Study the drawing (mm; zero at the part's minimum x, y, z) and answer. Give positions to 0.01 mm unless a question says otherwise; leave off trailing zeros. Order: outer loops, then holes, each group sorted by start corner. A loop starts at its lowest first (then second) coordinate and runs counter-clockwise, first axis right, second up. Notation, with made-up numbers: (17, 23) - (48, 23) arc R16 ccw to (48, 31) - close; hole circle Ø9 at (51.5, 58). An arc over 180 degrees is marked (long way). Put each result on its own line as item: value.
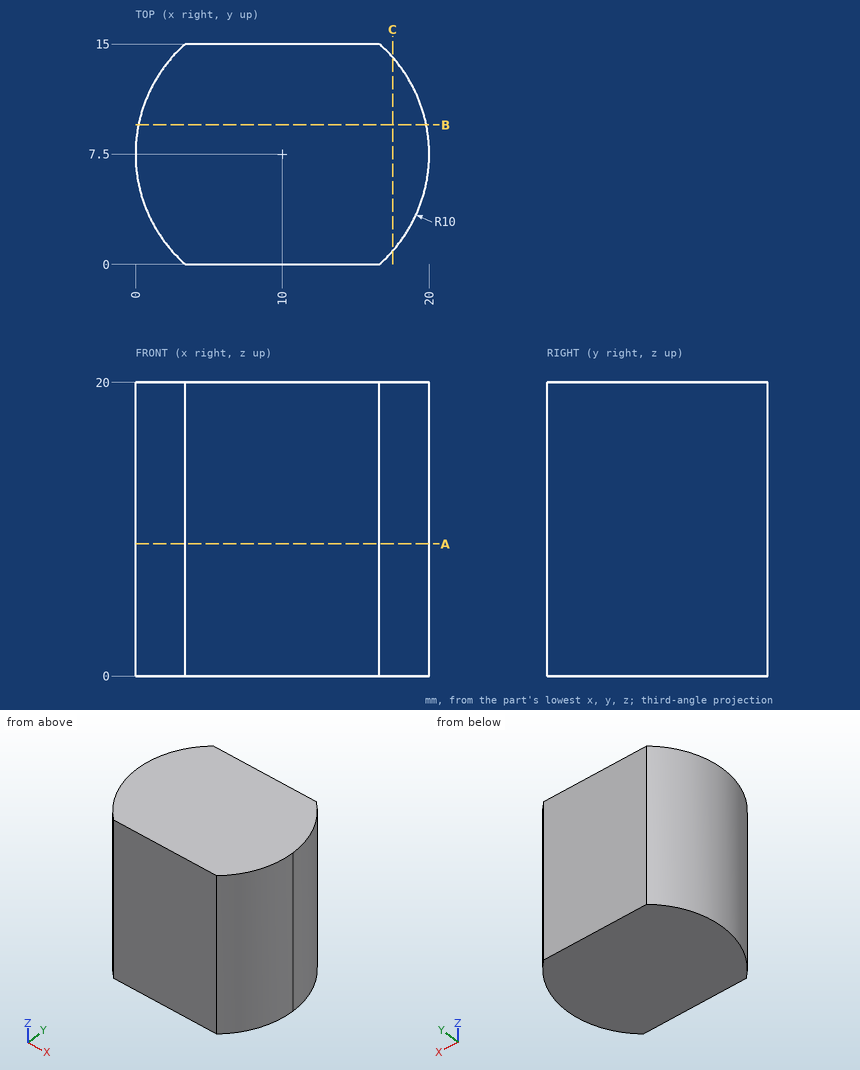
(1) Given pin 1 (5 mm diameter, centred on x = 8, y = 11.5, fed in from -Z); pin 2 (1 mm diameter, centred on y = 9.5, z = 18, fed in from -X); pin 3 (4 mm diameter, centred on y = 11, z = 5.5, fed in from +X); pin 4 (2 mm diameter, centred on y = 4.5, z = 10, fed in from +X), each flat-ended and moving along its own axis, determine where each tip first touches the part or whether it passes through.
Geometry check:
pin 1: stops at z = 0
pin 2: stops at x = 0.11
pin 3: stops at x = 19.89
pin 4: stops at x = 19.8
(2) Straight lines are drawn through the part: line 1 (X direction, y = 11.5, z = 16); line 2 (Y direction, x = 3.25, z = 9.25); line 3 (Y direction, x = 2.75, z = 11.25). For each, find the intervals that lie inside material, in ascending order.
Geometry check:
line 1: x = 0.83 to 19.17
line 2: y = 0.12 to 14.88
line 3: y = 0.61 to 14.39
(3) Section C-C, the plane x = 17.5 is taken. Write down the section's boundary in (y, z), then the cut area to 3 significant figures.
Geometry check:
outline: (0.89, 0) - (14.11, 0) - (14.11, 20) - (0.89, 20) - close
area: 265 mm²
(4) Section A-A, the plane z = 9 is taken. Write down the section's boundary in (x, y).
Geometry check:
outline: (3.39, 0) - (16.61, 0) arc R10 ccw to (20, 7.5) arc R10 ccw to (16.61, 15) - (3.39, 15) arc R10 ccw to start
(5) Section B-B, the plane y = 9.5 is taken. Write down the section's boundary in (x, z), then the cut area to 3 significant figures.
Geometry check:
outline: (0.2, 0) - (19.8, 0) - (19.8, 20) - (0.2, 20) - close
area: 392 mm²
